Answer from the drawing. Dimensions are ordinates in mm from the lowest x, y and z of the part. Give positions to 0.01 mm unless a question says otherwise; leave off trailing zeros. Order: outer loops, then holes, each group sorted by start corner. A loop starts at its lowest first (then second) coordinate and runs counter-clockwise, first axis right, second up. Notation, with made-up numbers: (64, -40) -> (87, -40) arc R14 cw to (87, -22) -> close; hole circle Ø9 at (-22.75, -27). An arc over 180 degrees is marked (long way). Answer as a JSON object with one key per item and string values. Group by question number.
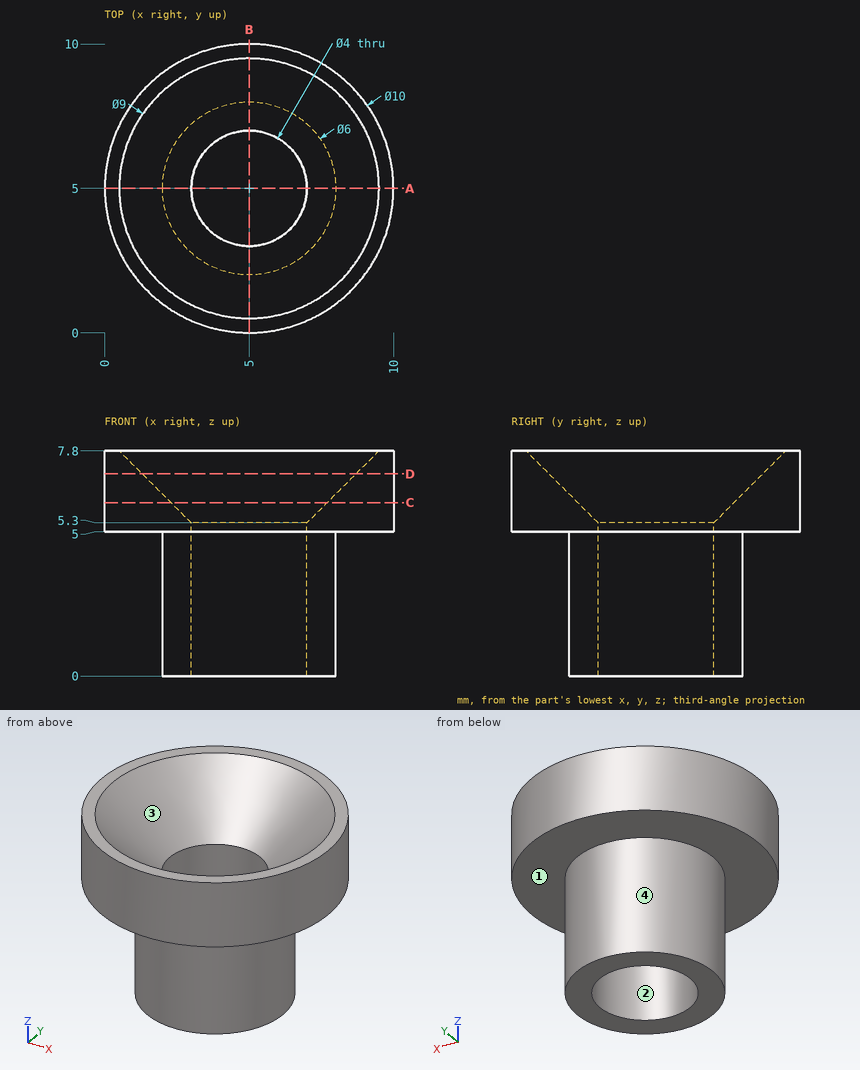
(1) Flat-ended cylindrical pins translate along their axes: pin 1 Ø2 at (y, z) = (4.5, 1) entering from -X; pin 2 Ø6 at (x, y) = (4, 5) entering from +Z. Find the tip coordinate at first contact, or state that the pin passes through.
(2) Find the intervals of material crossed by line 1 along Y through (x, z) = (5, 3.95); line 2 along Y through (x, z) = (3.75, 4.5); line 3 along X through (y, z) = (7.5, 6.25), in increasing order. Write a range as [from, to].
(3) A cutting plane is placed at C-C (z = 6). Determine the outline of the cut face in (x, y).
(4) A cutting plane is placed at D-D (z = 7). Determine the outline of the cut face in (x, y), and give its area (3 significant figures).
(5) A cutting plane is placed at A-A (y = 5). Determine the outline of the cut face in (x, z), and give its area (4 significant figures).
(6) For a pull along X with two mould halves and no side action, classify the marked faces 1, 2, 3 and 4 as +X half, -X half, draft (parallel to the pull), parting line (faces both ways), or undercut.
Check sheet entries:
{
 "1": {"pin 1": "stops at x = 2", "pin 2": "stops at z = 7.3"},
 "2": {"line 1": "y = [2, 3], [7, 8]", "line 2": "y = [2.27, 3.44], [6.56, 7.73]", "line 3": "x = [0.67, 3.43], [6.57, 9.33]"},
 "3": {"outline": "circle Ø10 at (5, 5); hole circle Ø5.4 at (5, 5)"},
 "4": {"outline": "circle Ø10 at (5, 5); hole circle Ø7.4 at (5, 5)", "area": "35.5 mm2"},
 "5": {"outline": "(0, 5) -> (2, 5) -> (2, 0) -> (3, 0) -> (3, 5.3) -> (0.5, 7.8) -> (0, 7.8) -> close; (7, 0) -> (8, 0) -> (8, 5) -> (10, 5) -> (10, 7.8) -> (9.5, 7.8) -> (7, 5.3) -> close", "area": "20.55 mm2"},
 "6": {"face 1": "draft", "face 2": "undercut", "face 3": "undercut", "face 4": "parting line"}
}
